Autodesk Fusion 360 part; units mm, degrees
sketch "saddle profile" plane through (0, 0, 0) normal (0, 0, 1) x (1, 0, 0) in component "hook"
  line L0 (0, 0) -> (0, 1.45)
  line L1 (0, 1.45) -> (4.9, 4)
  line L2 (4.9, 4) -> (11.5, 4)
  line L3 (11.5, 4) -> (11.5, 8)
  line L4 (11.5, 8) -> (37, 8)
  line L5 (37, 0) -> (0, 0)
  line L6 (37, 8) -> (37, 0) construction
  line L7 (74, 0) -> (74, 1.45)
  line L8 (74, 1.45) -> (69.1, 4)
  line L9 (69.1, 4) -> (62.5, 4)
  line L10 (62.5, 4) -> (62.5, 8)
  line L11 (62.5, 8) -> (37, 8)
  line L12 (37, 0) -> (74, 0)
  line L13 (0, 0) -> (0, -19.5) construction
  line L14 (0, -19.5) -> (74, -19.5) construction
  line L15 (74, -19.5) -> (74, 0) construction
  dimension "d7" = 1.45
  dimension "d8" = 6.6
  dimension "d9" = 4
  dimension "d10" = 11.5
  dimension "d11" = 4
  dimension "d12" = 37
  dimension "d13" = 19.5
sketch "mount profile" plane through (0, 0, 0) normal (0, 0, 1) x (1, 0, 0) in component "hook"
  line L0 (-11.6, 4.4845) -> (-11.6, -5)
  line L1 (0, -19.5) -> (74, -19.5)
  line L2 (-6.6, 1.45) -> (-0.1627, 4.8)
  line L3 (5.0442, 9.8) -> (-1.3859, 9.8)
  line L4 (-1.3859, 9.8) -> (-11.6, 4.4845)
  line L5 (-0.1627, 4.8) -> (5.0442, 4.8)
  line L6 (5.0442, 4.8) -> (5.0442, 9.8)
  line L7 (0, 1.45) -> (4.9, 4)
  line L8 (75.3859, 9.8) -> (72.2442, 9.8)
  line L9 (74.1627, 4.8) -> (67.2442, 4.8)
  line L10 (67.2442, 4.8) -> (72.2442, 9.8)
  line L11 (85.6, -5) -> (85.6, 4.4845)
  line L12 (80.6, 0) -> (-6.6, 0)
  line L13 (-6.6, 0) -> (-6.6, 1.45)
  line L14 (80.6, 0) -> (80.6, 1.45)
  line L15 (80.6, 1.45) -> (74.1627, 4.8)
  line L16 (-3.3814, 3.125) -> (-5.6896, 7.5603) construction
  line L17 (85.6, 4.4845) -> (75.3859, 9.8)
  line L18 (77.3814, 3.125) -> (79.6896, 7.5603) construction
  line L19 (85.6, 0.725) -> (80.6, 0.725) construction
  line L20 (-6.6, 0.725) -> (-11.6, 0.725) construction
  line L21 (85.6, -5) -> (74, -19.5)
  line L22 (-11.6, -5) -> (0, -19.5)
  line L23 (85.6, -5) -> (-11.6, -5) construction
  line L24 (37, 0) -> (37, -5) construction
  line L25 (74, -19.5) -> (74, -13.5)
  line L26 (74, -13.5) -> (0, -13.5)
  line L27 (0, -13.5) -> (0, -19.5)
  point P0 (74, 0)
  point P1 (74, -19.5)
  point P2 (0, -19.5)
  dimension "d16" = 74
  dimension "d17" = 1.45
  dimension "d19" = 4.8
  dimension "d20" = 62.2
  dimension "d22" = 6.6
  dimension "d23" = 45
  dimension "d24" = 6.6
  dimension "d25" = 5
  dimension "d26" = 19.5
  dimension "d29" = 6
  dimension "d47" = 5.2069
extrude "Extrude2" add sketch "mount profile" along normal blind 10 in component "hook"
sketch "mount" plane through (0, -19.5, 0) normal (0, -1, 0) x (1, 0, 0) in component "hook"
  line L0 (0, 0) -> (74, 0)
  line L1 (74, 0) -> (74, 10)
  line L2 (74, 10) -> (0, 10)
  line L3 (0, 10) -> (0, 0)
  line L4 (0, 0) -> (0, -12)
  line L5 (0, -12) -> (17, -20)
  line L6 (17, -20) -> (57, -20)
  line L7 (57, -20) -> (74, -12)
  line L8 (74, -12) -> (74, 0)
  circle A0 centre (24.6397, -10) radius 6.25 construction
  circle A1 centre (49.3603, -10) radius 6.25 construction
  circle A2 centre (24.6397, -10) radius 2.25
  circle A3 centre (49.3603, -10) radius 2.25
  line L9 (24.6397, -10) -> (49.3603, -10) construction
  line L10 (24.6397, -10) -> (0, -12) construction
  line L11 (49.3603, -10) -> (74, -12) construction
  line L12 (42, 0) -> (42, -20)
  line L13 (32, 0) -> (32, -20)
  line L14 (42, -3.75) -> (74, -3.75) construction
  line L15 (32, -3.75) -> (0, -3.75) construction
  dimension "d33" = 12.5
  dimension "d34" = 4.5
  dimension "d35" = 12
  dimension "d36" = 40
  dimension "d37" = 8
  dimension "d40" = 10
  dimension "d42" = 10
extrude "Extrude3" add sketch "mount" against normal blind 6 contours L0 L4 L5 L6 L13 | L0 L6 L12 L13 | L0 L6 L7 L8 L12 in component "hook"
extrude "Extrude4" add sketch "mount" against normal up to surface (13.5 mm away) from surface at -6 contours L0 L6 L12 L13 in component "hook"
chamfer "Chamfer1" distance 4 angle 45 2 edges at (47.2626, -13.5, -10.8136) (22.5419, -13.5, -10.8136) in component "hook"
chamfer "Chamfer2" distance 1 angle 45 47 edges at (74, -13.5, -6) (65.5, -13.5, -16) (49.5, -13.5, -20) (8.5, -13.5, -16) (24.5, -13.5, -20) (0, -13.5, -6) (42, 0, -10) (61.3, 0, 0) (12.7, 0, 0) (32, 0, -10) (37, 0, -20) (42, -6.75, -20) (32, -6.75, -20) (79.8, -12.25, 0) (79.8, -12.25, 10) (85.6, -0.2577, 10) (85.6, -0.2577, 0) (-5.8, -12.25, 0) (-5.8, -12.25, 10) (-11.6, -0.2577, 10) (-11.6, -0.2577, 0) (-6.493, 7.1423, 10) (-6.493, 7.1423, 0) (1.8291, 9.8, 0) (1.8291, 9.8, 10) (5.0442, 9.8, 5) (80.493, 7.1423, 0) (80.493, 7.1423, 10) (73.815, 9.8, 10) (73.815, 9.8, 0) (69.7442, 7.3, 10) (69.7442, 7.3, 0) (5.0442, 4.8, 5) (77.3814, 3.125, 0) (70.7035, 4.8, 0) (80.6, 0.725, 0) (2.4407, 4.8, 0) (-3.3814, 3.125, 0) (-6.6, 0.725, 0) (67.2442, 4.8, 5) (77.3814, 3.125, 10) (37, 0, 10) (80.6, 0.725, 10) (70.7035, 4.8, 10) (2.4407, 4.8, 10) (-3.3814, 3.125, 10) (-6.6, 0.725, 10) in component "hook"
component "hook" placed x (1, 0, 0) y (0, 1, 0) z (0, 0, 1) at (0, 0, 0)
equation "saddleW = 74 mm"
equation "saddleShelfD = 19.5 mm"
equation "saddleLipD = 11.5 mm"
equation "saddleLipT = 4 mm"
equation "saddleLipFlat = 6.6 mm"
equation "saddleEdgeH = 1.45 mm"
equation "d7 = saddleEdgeH"
equation "d8 = saddleLipFlat"
equation "d9 = saddleLipT"
equation "d10 = saddleLipD"
equation "d11 = d9"
equation "d12 = saddleW / 2"
equation "d13 = saddleShelfD"
equation "d16 = saddleW"
equation "d17 = saddleEdgeH"
equation "d19 = saddleLipT * 1.2"
equation "d20 = saddleW - ( 2 * saddleLipD ) + saddleLipFlat + 4.6 mm"
equation "d22 = saddleLipFlat"
equation "d24 = d22"
equation "d26 = saddleShelfD"
equation "mountT = 10 mm"
equation "d31 = mountT"
equation "d42 = mountT"
Source: CAD feature listing. Evaluate the final solid. Frame: model axes, mm. A direction names the side the tool comes from. Give positions to 0.01 mm unless a question says otherwise; leave off trailing zeros. Write each loop counter-clockwise with the first axis right and the second up, starting at its lowest first coordinate (ties: lowest second). Pieces come first, ordered by that corner, then holes. Notation, with made-up numbers: (61.25, -38) -> (112.25, -38) arc R7 ccw to (112.25, -27) -> close; hole circle Ø6 at (-6, -3.75). An arc over 180 degrees is marked (long way). Return JSON: item names as keys, results as strings. Group by question number.
1. Section D-D, the plane x = 8.5. Output: boundary loops of the cut face in (y, z).
2. Section C-C, the plane y = -2.25. Output: boundary loops of the cut face in (x, z).
3. Section A-A, the plane z = -10. Output: boundary loops of the cut face in (x, y), then the cut area to 3 significant figures.
4. Section B-B, the plane z = 2.5. Output: boundary loops of the cut face in (x, y), then the cut area to 3 significant figures.
5. Mould query, pull axis Z, two halves, no side actions, for faces 1 (the face through (80.34, 6.67, 9.49)), 2 (the face through (-5.5, -11.84, 0.51)), 3 (the face through (22.98, -18.51, -8.48)), 4 (the face through (1, 9.8, 5)). Classes: +Z half, -Z half, draft (parallel to the pull), parting line (faces both ways), or undercut.
6. Pin query (flat end, axial travel): pin 1 Ø8 at (x, y) = (19.5, 0) entering from -Z; pin 2 Ø3 at (x, y) = (74, -14.5) entering from -Z; pin 3 Ø15 at (x, z) = (63, -13.5) entering from +Y; pin 4 Ø4 at (x, z) = (49.36, -10) entering from -Y. Return the tip coordinate at first contact, or that it passes through.
7. Material intervals for line 1 (X direction, y = -18, z = -6); line 2 (Y direction, x = 64.5, z = 2.5); line 3 (Z direction, x = -0.5, y = -13.5), sorted ascending. Write a range as from..to.
8. Access query for faces 5 (the face through (-3.43, 3.1, 4.94)), 6 (the face through (5.044, 7, 5)), 7 (the face through (77.82, 3.45, 0.51)). Directions: +Z, -Z, +X, -X, +Y, -Y. A direction counts if a zero-diameter tool reaches every point of the face in a straight line with its end or side. Return the directions, or none.
Determined:
{
 "1": {"outline": "(-19.5, -16) -> (-14.5, -16) -> (-13.5, -14.89) -> (-13.5, 0) -> (-1, 0) -> (0, 1) -> (0, 9) -> (-1, 10) -> (-19.5, 10) -> close"},
 "2": {"outline": "(-11.6, 1) -> (-10.6, 0) -> (32, 0) -> (32, -19) -> (33, -20) -> (41, -20) -> (42, -19) -> (42, 0) -> (84.6, 0) -> (85.6, 1) -> (85.6, 9) -> (84.6, 10) -> (-10.6, 10) -> (-11.6, 9) -> close"},
 "3": {"outline": "(0, -19.5) -> (22.39, -19.5) -> (22.39, -17.5) -> (18.39, -13.5) -> (1, -13.5) -> (0, -14.5) -> close; (26.89, -19.5) -> (47.11, -19.5) -> (47.11, -17.5) -> (43.11, -13.5) -> (42, -13.5) -> (42, -1) -> (41, 0) -> (33, 0) -> (32, -1) -> (32, -13.5) -> (30.89, -13.5) -> (26.89, -17.5) -> close; (51.61, -19.5) -> (74, -19.5) -> (74, -14.5) -> (73, -13.5) -> (55.61, -13.5) -> (51.61, -17.5) -> close", "area": "491 mm2"},
 "4": {"outline": "(-11.6, -5) -> (0, -19.5) -> (74, -19.5) -> (85.6, -5) -> (85.6, 4.48) -> (75.39, 9.8) -> (72.24, 9.8) -> (67.95, 5.51) -> (68.24, 4.8) -> (74.16, 4.8) -> (80.6, 1.45) -> (80.6, 0) -> (-6.6, 0) -> (-6.6, 1.45) -> (-0.16, 4.8) -> (4.04, 4.8) -> (5.04, 5.8) -> (5.04, 8.8) -> (4.04, 9.8) -> (-1.39, 9.8) -> (-11.6, 4.48) -> close", "area": "1,900 mm2"},
 "5": {"face 1": "+Z half", "face 2": "-Z half", "face 3": "undercut", "face 4": "draft"},
 "6": {"pin 1": "stops at z = 0", "pin 2": "stops at z = -12.71", "pin 3": "stops at y = -13.5", "pin 4": "passes through"},
 "7": {"line 1": "x = 0..74", "line 2": "y = -19.5..0", "line 3": "z = 0..10"},
 "8": {"face 5": "+Z, -Z", "face 6": "+Z, -Z, +Y", "face 7": "-Z"}
}
